from build123d import *

# Parameters (mm, degrees)
SKETCH1_R           = 4
BOSS_EXTRUDE1_DEPTH = 30
CUT_EXTRUDE3_START  = -15
CUT_EXTRUDE3_DEPTH  = 15
ECHELLE1_SCALE      = 0.6


with BuildPart() as part:
    # Sketch1 → Boss-Extrude1 (new body)
    with BuildSketch(Plane.XY):
        with BuildLine():
            Line((0, -10), (60, -10))
            Line((60, -10), (60, 50))
            ThreePointArc((60, 50), (50, 60), (40, 50))
            Line((40, 50), (0, 10))
            ThreePointArc((0, 10), (-10, 0), (0, -10))
        make_face()
        with Locations((50, 50)):
            Circle(SKETCH1_R, mode=Mode.SUBTRACT)
        Circle(SKETCH1_R, mode=Mode.SUBTRACT)
    extrude(amount=BOSS_EXTRUDE1_DEPTH)

    # Sketch3 → Cut-Extrude3 (cut)
    with BuildSketch(Plane.XY.offset(30).offset(CUT_EXTRUDE3_START)):
        with BuildLine():
            Line((60, -217.989898732), (60, -10))
            Line((60, -10), (60, 50))
            ThreePointArc((60, 50), (50, 60), (40, 50))
            Line((40, 50), (0, 10))
            ThreePointArc((0, 10), (-10, 0), (0, -10))
            Line((0, -10), (60, -10))
            Line((60, -10), (25, -10))
            Line((25, -10), (25, 35))
            Line((25, 35), (25, 242.989898732))
            Line((25, 242.989898732), (-389.785969286, 211.497176047))
            Line((-389.785969286, 211.497176047), (-354.785969286, -249.482621417))
            Line((-354.785969286, -249.482621417), (60, -217.989898732))
        make_face()
    extrude(amount=CUT_EXTRUDE3_DEPTH, mode=Mode.SUBTRACT)


with BuildPart() as part_1:
    # Echelle1: scaled about (37.827967632, 17.936559761, 13.650169575)
    add(part.part.scale(ECHELLE1_SCALE).moved(Location((15.131187053, 7.174623904, 5.46006783))))


solid = part_1.part
Check sheet for the modelled part. Datum: model origin and axes. Units: mm. A direction names the side the tool comes from. Round coordinates to 2 decimals unless told otherwise and drop trailing zeros. Loops run counter-clockwise (first coordinate to the right, second up) from the corner with the lowest first, then second, coordinate; pieces in that order, holes last. Notation, with made-up numbers: M 9.5,-23 L 64.5,-23 A25 cw 64.5,-7 Z; hole C 68.25,-12 d10. An arc over 180 degrees is marked long. One line per item, written item: value.
(1) Depth check by flat-ended pin: pin 1 Ø1 at (x, z) = (43.5, 21.5) entering from +Y; pin 2 Ø2 at (x, z) = (38, 11) entering from +Y; pin 3 Ø2.5 at (y, z) = (16, 19.5) entering from -X. Enter the tip coordinate at first touch or a pass-through.
Computed values:
pin 1: stops at y = 43.07
pin 2: stops at y = 37.04
pin 3: stops at x = 30.13
(2) Release check for a two-part mould opening along Y. For faces 3 (the face through (40, 18, 23.46)), 4 (the face through (44.61, 34.83, 14.33)), 5 (the face through (9.133, 7.307, 9.897)) record: +Y half, -Y half, draft (parallel to the pull), parting line (faces both ways), or undercut.
Computed values:
face 3: draft
face 4: undercut
face 5: parting line
(3) Sectioned sample at A-A, the plane z = 21. Record the cut outline in (x, y).
Computed values:
outline: M 30.13,1.17 L 51.13,1.17 L 51.13,37.17 A6 ccw 39.13,37.17 L 30.13,28.17 Z; hole C 45.13,37.17 d4.8
(4) Access from +Z, -Z, +X, -X, +Y, -Y to the whole of each face (thin tool, end or side, straight path). Record for faces 1 (the face through (30.131, 14, 19)), 2 (the face through (51.131, 19, 14)).
Computed values:
face 1: +Z, -X, +Y, -Y
face 2: +Z, -Z, +X, +Y, -Y
(5) Thickness scan on line 1 (X direction, y = 8, z = 16.5); line 2 (Z direction, x = 25.5, y = 7); line 3 (X direction, y = 38, z = 12.5). Record the ranges inside material, lowest first.
Computed values:
line 1: x = 30.13 to 51.13
line 2: z = 5.46 to 14.46
line 3: x = 39.19 to 42.88, 47.38 to 51.07
(6) Sectioned sample at D-D, the plane z = 10. Record the cut outline in (x, y).
Computed values:
outline: M 15.13,1.17 L 51.13,1.17 L 51.13,37.17 A6 ccw 39.13,37.17 L 15.13,13.17 A6 ccw Z; hole C 15.13,7.17 d4.8; hole C 45.13,37.17 d4.8
(7) Sectioned sample at B-B, the plane x = 44.5. Record the cut outline in (y, z), then the cut area to 3 significant figures.
Computed values:
outline: M 1.17,5.46 L 34.86,5.46 L 34.86,23.46 L 1.17,23.46 Z; M 39.49,5.46 L 43.14,5.46 L 43.14,23.46 L 39.49,23.46 Z
area: 672 mm^2
(8) Sectioned sample at C-C, the plane y = 8.5. Record the cut outline in (x, z), then the cut area to 3 significant figures.
Computed values:
outline: M 9.28,5.46 L 13.13,5.46 L 13.13,14.46 L 9.28,14.46 Z; M 17.13,5.46 L 51.13,5.46 L 51.13,23.46 L 30.13,23.46 L 30.13,14.46 L 17.13,14.46 Z
area: 530 mm^2
